Read the model definition and answer for the solid it produces. Units are mm, in the model's axes. Face numbers are marked on the shaded views. A direction names the side the tool comes from. Coordinates: 2 decimals unless noted, no trailing zeros. Loops run counter-clockwise (first coordinate to the right, second up) from the corner with the lowest first, then second, coordinate; pieces in that order, holes last.
Autodesk Inventor part; units mm, degrees
ref_plane "YZ Plane" through (0, 0, 0) normal (1, 0, 0) x (0, 1, 0)
ref_plane "XZ Plane" through (0, 0, 0) normal (0, 1, 0) x (-1, 0, 0)
ref_plane "XY Plane" through (0, 0, 0) normal (0, 0, 1) x (1, 0, 0)
sketch "Sketch1" plane through (0, 0, 0) normal (0, 0, 1) x (1, 0, 0)
  line L0 (10, 11) -> (-10, 11)
  line L1 (-10, 11) -> (-10, -11)
  line L2 (-10, -11) -> (10, -11)
  line L3 (10, -11) -> (10, 11)
  line L4 (10, 11) -> (-10, -11) construction
  line L5 (-10, 11) -> (10, -11) construction
  line L6 (0, -12.7143) -> (0, 12.7143) construction
  line L7 (12, 0) -> (-13.2325, 0) construction
  point P0 (0, 0)
  dimension "d0" = 20
  dimension "d1" = 22
extrude "Extrusion1" add sketch "Sketch1" along normal blind 5
chamfer "Chamfer7" distance 3 angle 45 2 edges at (10, 0, 5) (-10, 0, 5)
sketch "Sketch2" plane through (0, 0, 0) normal (0, 0, -1) x (-1, 0, 0)
  line L0 (2, 1.1547) -> (2, -1.1547)
  line L1 (2, -1.1547) -> (0, -2.3094)
  line L2 (0, -2.3094) -> (-2, -1.1547)
  line L3 (-2, -1.1547) -> (-2, 1.1547)
  line L4 (-2, 1.1547) -> (0, 2.3094)
  line L5 (0, 2.3094) -> (2, 1.1547)
  line L6 (10, -11) -> (-10, -11)
  line L7 (-2.75, 11) -> (2.75, 11)
  line L8 (2.75, 11) -> (2.75, -11)
  line L9 (2.75, -11) -> (-2.75, -11)
  line L10 (-2.75, -11) -> (-2.75, 11)
  line L11 (-2.75, 11) -> (2.75, -11) construction
  line L12 (2.75, 11) -> (-2.75, -11) construction
  point P0 (0, 0)
  dimension "d5" = 5.5
extrude "Extrusion2" add sketch "Sketch2" along normal blind 1
sketch "Sketch3" plane through (0, 0, -1) normal (0, 0, -1) x (-1, 0, 0)
  line L0 (2, -1.1547) -> (0, -2.3094)
  line L1 (0, -2.3094) -> (-2, -1.1547)
  line L2 (-2, -1.1547) -> (-2, 1.1547)
  line L3 (-2, 1.1547) -> (0, 2.3094)
  line L4 (0, 2.3094) -> (2, 1.1547)
  line L5 (2, 1.1547) -> (2, -1.1547)
  line L6 (-2.75, 2.75) -> (2.75, 2.75)
  line L7 (2.75, 2.75) -> (2.75, -2.75)
  line L8 (2.75, -2.75) -> (-2.75, -2.75)
  line L9 (-2.75, -2.75) -> (-2.75, 2.75)
  line L10 (-2.75, 2.75) -> (2.75, -2.75) construction
  line L11 (2.75, 2.75) -> (-2.75, -2.75) construction
  point P0 (0, 0)
  dimension "d8" = 5.5
  dimension "d9" = 5.5
extrude "Extrusion3" cut sketch "Sketch3" against normal up to surface (1 mm away) from surface at 0
sketch "Sketch8" plane through (0, 0, 5) normal (0, 0, 1) x (1, 0, 0)
  line L0 (-7, -11) -> (7, -11)
  line L1 (7, 11) -> (-7, 11)
  line L2 (-1.5, -11) -> (1.5, -11)
  line L3 (1.5, -11) -> (1.5, -4.4105)
  line L4 (1.5, -4.4105) -> (-1.5, -4.4105)
  line L5 (-1.5, -4.4105) -> (-1.5, -11)
  line L6 (-1.5, 11) -> (1.5, 11)
  line L7 (1.5, 11) -> (1.5, 4.4105)
  line L8 (1.5, 4.4105) -> (-1.5, 4.4105)
  line L9 (-1.5, 4.4105) -> (-1.5, 11)
  line L10 (-1.5, -11) -> (-1.5, 11) construction
  line L11 (1.5, -11) -> (1.5, 11) construction
  line L12 (1.5, 4.4105) -> (0, 0) construction
  line L13 (0, 0) -> (-1.5, 4.4105) construction
  line L14 (1.5, -4.4105) -> (0, 0) construction
  line L15 (-1.5, -4.4105) -> (0, 0) construction
  dimension "d83" = 3
extrude "Extrusion7" cut sketch "Sketch8" against normal blind 3
chamfer "Chamfer8" distance 3 angle 45 4 edges at (-1.5, 7.7052, 5) (-1.5, -7.7052, 5) (1.5, -7.7052, 5) (1.5, 7.7052, 5)
sketch "Sketch9" plane through (10, -11, 0) normal (1, 0, 0) x (0, 0, -1)
  line L0 (-2, 0) -> (-2, 22) construction
  line L1 (-1, -1) -> (-1, 22.6316) construction
  line L2 (-1, 1.0298) -> (-4, 1.0298)
  line L3 (-4, 1.0298) -> (-4, 6.5895)
  line L4 (-4, 6.5895) -> (-1, 6.5895)
  line L5 (-1, 6.5895) -> (-1, 1.0298)
  line L6 (-1, 20.9702) -> (-4, 20.9702)
  line L7 (-4, 20.9702) -> (-4, 15.4105)
  line L8 (-4, 15.4105) -> (-1, 15.4105)
  line L9 (-1, 15.4105) -> (-1, 20.9702)
  line L10 (-5, 6.5895) -> (-2, 6.5895) construction
  line L11 (-2, 15.4105) -> (-5, 15.4105) construction
  point P0 (0, 11)
  dimension "d85" = 1
extrude "Extrusion8" cut sketch "Sketch9" against normal through all
sketch "Sketch10" plane through (0, 0, 5) normal (0, 0, 1) x (1, 0, 0)
  point P0 (0, 0)
  point P1 (0, 0)
hole "Hole2" at (0, 0, 5) direction (0, 0, -1) diameter 4.5 end through all counterbore diameter 8 counterbore depth 2
properties part number "harness clip"
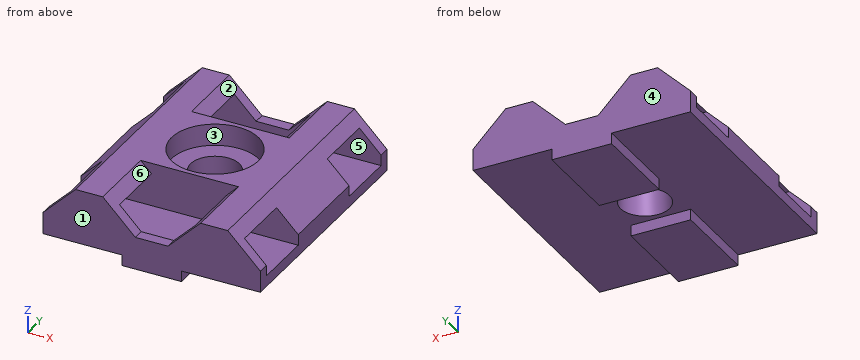
Q1. A cutting plane is placed at A-A (y = 5.5). Give the vertices of the cut face in (x, z), then the cut area to 3 significant figures.
Findings below:
outline: (-10, 0) - (-2.75, 0) - (-2.75, -1) - (2.75, -1) - (2.75, 0) - (10, 0) - (10, 1) - (-10, 1) - close; (-8, 4) - (-3.5, 4) - (-4.5, 5) - (-7, 5) - close; (3.5, 4) - (8, 4) - (7, 5) - (4.5, 5) - close
area: 32.5 mm2
Q2. Straight lines are drawn through the part: probe 1 along Y at (x, z) = (5, 3.75); probe 2 along Y at (x, z) = (0, 1.25); probe 3 along X at (y, z) = (0, 1). For each, find the intervals that lie inside material, in ascending order.
Findings below:
probe 1: y = -11 to -9.97, -4.41 to 4.41, 9.97 to 11
probe 2: y = -11 to -9.97, -4.41 to -2.25, 2.25 to 4.41, 9.97 to 11
probe 3: x = -10 to -2.25, 2.25 to 10
Q3. A cutting plane is placed at B-B (x = 0). Give the vertices of the cut face in (y, z).
Findings below:
outline: (-11, -1) - (-2.75, -1) - (-2.75, 0) - (-2.25, 0) - (-2.25, 3) - (-4, 3) - (-4, 5) - (-4.41, 5) - (-4.41, 1) - (-9.97, 1) - (-9.97, 2) - (-11, 2) - close; (2.25, 0) - (2.75, 0) - (2.75, -1) - (11, -1) - (11, 2) - (9.97, 2) - (9.97, 1) - (4.41, 1) - (4.41, 5) - (4, 5) - (4, 3) - (2.25, 3) - close
Q4. A cutting plane is placed at D-D (x = 7.25). Give the vertices of the cut face in (y, z), then the cut area to 3 significant figures.
Findings below:
outline: (-11, 0) - (11, 0) - (11, 4.75) - (-11, 4.75) - close; hole (-9.97, 1) - (-4.41, 1) - (-4.41, 4) - (-9.97, 4) - close; hole (4.41, 1) - (9.97, 1) - (9.97, 4) - (4.41, 4) - close
area: 71.1 mm2
Q5. Which of the six approach directions +Z, -Z, +X, -X, +Y, -Y give full straight-line access (tool end or side, diameter ignored) to the marked faces 4, 5 and 6?
Findings below:
face 4: +Z, -Z, +X, -X, +Y
face 5: +X, -X
face 6: +Z, -Y
Q6. Flat-ended cylindrical pins translate along their axes: pin 1 Ø0.8 at (y, z) = (8.5, -0.5) entering from -X; pin 2 Ø1.5 at (x, y) = (-3, -1) entering from -Z; pin 3 Ø2.5 at (x, y) = (0, 0) entering from -Z. Find the tip coordinate at first contact, or state that the pin passes through.
Findings below:
pin 1: stops at x = -2.75
pin 2: stops at z = 0
pin 3: passes through
Q7. Determine the mould class of the marked faces 1, 2 and 3 for opening direction Y: +Y half, -Y half, draft (parallel to the pull), parting line (faces both ways), or undercut.
Findings below:
face 1: -Y half
face 2: draft
face 3: undercut
Q8. A cutting plane is placed at C-C (z = 2.25). Give the vertices of the cut face in (x, y), then the cut area to 3 significant figures.
Findings below:
outline: (-9.75, -11) - (-1.75, -11) - (-1.75, -9.97) - (-9.75, -9.97) - close; (-9.75, -4.41) - (9.75, -4.41) - (9.75, 4.41) - (-9.75, 4.41) - close; (-9.75, 9.97) - (-1.75, 9.97) - (-1.75, 11) - (-9.75, 11) - close; (1.75, -11) - (9.75, -11) - (9.75, -9.97) - (1.75, -9.97) - close; (1.75, 9.97) - (9.75, 9.97) - (9.75, 11) - (1.75, 11) - close; hole circle Ø4.5 at (0, 0)
area: 189 mm2
